Autodesk Inventor part; units mm, degrees
ref_plane "YZ Plane" through (0, 0, 0) normal (1, 0, 0) x (0, 1, 0)
ref_plane "XZ Plane" through (0, 0, 0) normal (0, 1, 0) x (-1, 0, 0)
ref_plane "XY Plane" through (0, 0, 0) normal (0, 0, 1) x (1, 0, 0)
sketch "스케치1" plane through (0, 0, 0) normal (0, 0, 1) x (1, 0, 0)
  circle A0 centre (0, 0) radius 4.1
  circle A1 centre (0, 0) radius 1
  dimension "d0" = 8.2
extrude "돌출1" add sketch "스케치1" along normal blind 8.62
sketch "스케치2" plane through (0, 0, 8.62) normal (0, 0, 1) x (1, 0, 0)
  circle A0 centre (0, 0) radius 17
  circle A1 centre (0, 0) radius 4.1
  dimension "d3" = 34
extrude "돌출2" add sketch "스케치2" against normal blind 6.6
sketch "스케치3" plane through (0, 0, 8.62) normal (0, 0, 1) x (1, 0, 0)
  point P0 (0, 0)
sketch "스케치4" plane through (0, 0, 8.62) normal (0, 0, 1) x (1, 0, 0)
  circle A0 centre (0, 0) radius 17
  circle A1 centre (0, 0) radius 1
  circle A2 centre (0, 0) radius 14
  dimension "d6" = 3
extrude "돌출3" cut sketch "스케치4" against normal blind 0.5 contours A0
sketch "스케치5" plane through (0, 0, 2.02) normal (0, 0, -1) x (-1, 0, 0)
  circle A0 centre (0, 0) radius 4.1
  circle A1 centre (0, 0) radius 17
  circle A2 centre (0, 0) radius 14
extrude "돌출4" cut sketch "스케치5" against normal blind 0.5 contours A1
fillet "모깎기1" radius 2 2 edges at (-17, 0, 2.52) (-17, 0, 8.12)
sketch "스케치6" plane through (0, 0, 8.62) normal (0, 0, 1) x (1, 0, 0)
  circle A0 centre (0, 0) radius 14
  circle A1 centre (0, 0) radius 1
  circle A2 centre (0, 0) radius 14
  circle A3 centre (0, 0) radius 14
  line L0 (0, 0) -> (1, 0) construction
  line L1 (0, 0) -> (-0.5, -0.866)
  line L2 (2.026, -1.5128) -> (9.8898, -1.5625)
  line L3 (0.866, -1.5) -> (0.8629, -1.5055)
  line L4 (-2.3094, -1) -> (-6.2488, -7.8232)
  line L5 (13.9097, -1.5879) -> (13.9902, -1.5884)
  line L6 (0.296, 2.4873) -> (-3.6507, 9.3232)
  line L7 (-2.3094, 1) -> (-6.2488, 7.8232)
  line L8 (-8.2587, 11.3046) -> (-8.299, 11.3744)
  line L9 (-5.6607, 12.8046) -> (-5.701, 12.8744)
  arc A4 (-2.2841, -12.2895) -> (11.7585, -4.2411) centre (0, 0) ccw
  line L10 (0, 0) -> (1, -0.0063)
  line L11 (0.2813, -2.5128) -> (-3.6507, -9.3232)
  line L12 (-5.6607, -12.8046) -> (-5.701, -12.8744)
  line L13 (0, 0) -> (-0.5, 0.866)
  line L14 (2.0154, 1.4873) -> (9.9088, 1.4374)
  line L15 (13.9286, 1.412) -> (14.0092, 1.4115)
  arc A5 (11.8112, 4.0921) -> (-2.2841, 12.2895) centre (0, 0) ccw
  arc A6 (-9.501, 8.1229) -> (-9.501, -8.1229) centre (0, 0) ccw
  line L16 (0, 0) -> (1, 0) construction
  arc A7 (9.9088, 1.4374) -> (11.8112, 4.0921) centre (9.9214, 3.4374) ccw
  arc A8 (-2.2841, 12.2895) -> (-3.6507, 9.3232) centre (-1.9187, 10.3232) ccw
  arc A9 (0.296, 2.4873) -> (2.0154, 1.4873) centre (2.0281, 3.4873) ccw
  arc A10 (2.026, -1.5128) -> (0.2813, -2.5128) centre (2.0133, -3.5128) ccw
  arc A11 (11.7585, -4.2411) -> (9.8898, -1.5625) centre (9.8772, -3.5625) ccw
  arc A12 (-3.6507, -9.3232) -> (-2.2841, -12.2895) centre (-1.9187, -10.3232) ccw
  arc A13 (-9.501, -8.1229) -> (-6.2488, -7.8232) centre (-7.9808, -6.8232) ccw
  arc A14 (-6.2488, 7.8232) -> (-9.501, 8.1229) centre (-7.9808, 6.8232) ccw
  arc A15 (-2.3094, -1) -> (-2.3094, 1) centre (-4.0415, 0) ccw
  point P0 (12.4189, 1.4215)
  point P1 (12.3999, -1.5784)
  point P2 (-4.9058, -11.4971)
  point P3 (-7.5039, -9.9971)
  point P4 (-7.5039, 9.9971)
  point P5 (-4.9058, 11.4971)
  dimension "d26" = 1.5
  dimension "d28" = 1.5
  dimension "d29" = 2
extrude "돌출5" cut sketch "스케치6" against normal up to next contours L2 A11 A4 A12 L11 A10 | L4 A13 A6 A14 L7 A15 | L6 A8 A5 A7 L14 A9
properties part number "n2_miniWheel"
Can you work these out from the model? Positions are in its coordinate system, mm. Give positions to 0.01 mm unless a question says otherwise; leave off trailing zeros. Write each loop counter-clockwise with the first axis right and the second up, starting at its lowest first coordinate (ties: lowest second). Pieces come first, ordered by that corner, then holes. Notation, with made-up numbers: (-14.5, -16.75) -> (8.5, -16.75) arc R29 ccw to (8.5, 17.25) -> close; hole circle Ø1 at (0.5, -26.5). An arc over 180 degrees is marked (long way). Answer as a JSON object with one key per item and string values. Group by question number.
Item 1: We'd pull the mould along X, two halves only. Please class faces 1 (the face through (1.01, 1.766, 4.37)), 2 (the face through (-2.07, 3.54, 1)), 3 (the face through (3, 0, 8.62)): +X half, -X half, draft (parallel to the pull), parting line (faces both ways), or undercut.
Item 2: Suppose I cut it at D-D (x = 5.5). State how many separate pieces and enclosed holes the cut face has, plus the area to 3 significant figures.
Item 3: I'm going to push flat-ended pins straight in: P1, Ø3, axis at y = -11, z = 5.5, coming from the +X side; P2, Ø3, axis at y = 9, z = 7, coming from the -X side. Where does each tip first touch, or does it pass through?
Item 4: Suppose I cut it at C-C (z = 3.75). Please give me the cut outline in (x, y).
Item 5: Suppose I cut it at B-B (z = 1.25). Please give me the cut outline in (x, y), plus the area to 3 significant figures.
Item 6: Suppose I cut it at A-A (y = 0). Please give me the cut outline in (x, z).
Item 7: Please list where these lines run through material, in increasing order: line 1 (Y direction, x = -1.5, z = 3.25); line 2 (X direction, y = -7.5, z = 3.75); line 3 (Y direction, x = 10, z = 7). Write a range as [from, to].
Findings:
{
 "1": {"face 1": "undercut", "face 2": "-X half", "face 3": "draft"},
 "2": {"separate pieces": "3", "enclosed holes": "0", "area": "73.9 mm²"},
 "3": {"P1": "stops at x = 14.1", "P2": "stops at x = -15.17"},
 "4": {"outline": "circle Ø33.69 at (0, 0); hole (-9.5, -8.12) arc R2 ccw to (-6.25, -7.82) -> (-2.31, -1) arc R2 ccw to (-2.31, 1) -> (-6.25, 7.82) arc R2 ccw to (-9.5, 8.12) arc R12.5 ccw to start; hole (-3.65, -9.32) arc R2 ccw to (-2.28, -12.29) arc R12.5 ccw to (11.76, -4.24) arc R2 ccw to (9.89, -1.56) -> (2.03, -1.51) arc R2 ccw to (0.28, -2.51) -> close; hole (-3.65, 9.32) -> (0.3, 2.49) arc R2 ccw to (2.02, 1.49) -> (9.91, 1.44) arc R2 ccw to (11.81, 4.09) arc R12.5 ccw to (-2.28, 12.29) arc R2 ccw to start; hole circle Ø2 at (0, 0)"},
 "5": {"outline": "(-3.21, -2.55) arc R4.1 ccw to (-0.61, -4.05) -> (0.28, -2.51) arc R2 cw to (2.03, -1.51) -> (3.81, -1.52) arc R4.1 ccw to (3.83, 1.48) -> (2.02, 1.49) arc R2 cw to (0.3, 2.49) -> (-0.61, 4.05) arc R4.1 ccw to (-3.21, 2.55) -> (-2.31, 1) arc R2 cw to (-2.31, -1) -> close; hole circle Ø2 at (0, 0)", "area": "29.7 mm²"},
 "6": {"outline": "(-17, 4.52) arc R2 ccw to (-15, 2.52) -> (-14, 2.52) -> (-14, 2.02) -> (-12.5, 2.02) -> (-12.5, 8.62) -> (-14, 8.62) -> (-14, 8.12) -> (-15, 8.12) arc R2 ccw to (-17, 6.12) -> close; (-2.04, 0) -> (-1, 0) -> (-1, 8.62) -> (-2.04, 8.62) -> close; (1, 0) -> (4.1, 0) -> (4.1, 2.02) -> (14, 2.02) -> (14, 2.52) -> (15, 2.52) arc R2 ccw to (17, 4.52) -> (17, 6.12) arc R2 ccw to (15, 8.12) -> (14, 8.12) -> (14, 8.62) -> (1, 8.62) -> close"},
 "7": {"line 1": "y = [-16.48, -12.41], [-5.6, 5.6], [12.41, 16.48]", "line 2": "x = [-15.08, -10], [-6.06, -2.6], [10, 15.08]", "line 3": "y = [-13.49, -7.5], [-1.57, 1.44], [7.5, 13.49]"}
}
